Geometry: final body of the model. Coordinates: model frame, mm. Face numbers are marked on the shaded views. A direction names the side the tool comes from. Round coordinates to 2 decimals unless told otherwise and drop trailing zeros. Write each loop counter-clockwise with the first axis right and the second up, starting at its lowest first coordinate (ties: lowest second). Pieces come first, ordered by that corner, then holes.
from build123d import *

# Parameters (mm, degrees)
F0_W     = 12.7
F0_H     = 25.4
F1_DEPTH = 25.4
F3_W     = 12.7
F3_H     = 12.7
F4_DEPTH = 6.35
F5_W     = 12.7
F5_H     = 25.4
F6_DEPTH = 12.7


with BuildPart() as f1:
    # F0 (on Front) → F1 (new body)
    with BuildSketch(Plane.XZ):
        with Locations((6.35, 12.7)):
            Rectangle(F0_W, F0_H)
    extrude(amount=-F1_DEPTH)

    # F3 (on face) → F4 (cut)
    with BuildSketch(Plane.XZ):
        with Locations((6.35, 12.7)):
            Rectangle(F3_W, F3_H)
    extrude(amount=-F4_DEPTH, mode=Mode.SUBTRACT)

    # F5 (on face) → F6 (join)
    with BuildSketch(Plane.YZ.offset(12.7)):
        with Locations((19.05, 12.7)):
            Rectangle(F5_W, F5_H)
    extrude(amount=F6_DEPTH)


solid = f1.part
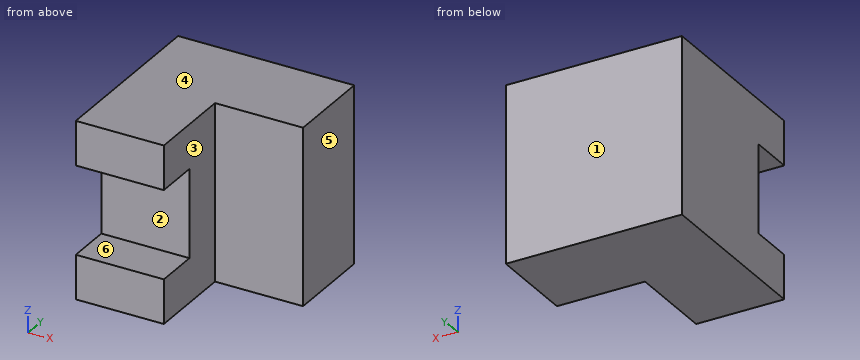
1) Section D-D on y = 12.25. Output: boundary loops of the cut face in (x, z).
2) First-contact query: P1, Ø10, axis at x = 14.5, y = 18, coming from the -Z side; P2, Ø2, axis at x = 17.5, z = 14.5, coming from the -Y side; P3, Ø6.5, axis at y = 4.5, z = 16, coming from the +X side; P4, Ø6.5, axis at x = 9.5, z = 15, coming from the -Y side. Flat tips, straight axial feed; report the tip coordinate or a pass-through.
3) Section C-C on z = 3.75. Output: boundary loops of the cut face in (x, y), plus the area to 3 significant figures.
4) Draft query along Z for the marked faces 4, 5 and 6. Return one class per face: pulls with the +Z half, pulls with the -Z half, needs draft (parallel to the pull), parting line crosses it, or undercut.
5) Line query: probe 1 along Z at (x, y) = (4, 3.5); probe 2 along Y at (x, z) = (6.25, 8); probe 3 along Y at (x, z) = (18.5, 3). Output: solid intervals per line, ascending.
6) Section B-B on x = 11.5. Output: boundary loops of the cut face in (y, z), plus the area to 3 significant figures.
7) Section A-A on y = 2. Output: boundary loops of the cut face in (x, z).
8) Reachability of the marked faces 1, 2 and 3 from +Z, -Z, +X, -X, +Y, -Y: full face, straight path, thin tool, end or side. Return the list, or none.
Filled in:
1. outline: (0, 0) - (12.7, 0) - (12.7, 25.4) - (0, 25.4) - close
2. P1: stops at z = 0
2. P2: stops at y = 12.7
2. P3: stops at x = 12.7
2. P4: stops at y = 6.35
3. outline: (0, 0) - (12.7, 0) - (12.7, 12.7) - (25.4, 12.7) - (25.4, 25.4) - (0, 25.4) - close
3. area: 484 mm2
4. face 4: pulls with the +Z half
4. face 5: needs draft
4. face 6: undercut
5. probe 1: z = 0 to 6.35, 19.05 to 25.4
5. probe 2: y = 6.35 to 25.4
5. probe 3: y = 12.7 to 25.4
6. outline: (0, 0) - (25.4, 0) - (25.4, 25.4) - (0, 25.4) - (0, 19.05) - (6.35, 19.05) - (6.35, 6.35) - (0, 6.35) - close
6. area: 565 mm2
7. outline: (0, 0) - (12.7, 0) - (12.7, 6.35) - (0, 6.35) - close; (0, 19.05) - (12.7, 19.05) - (12.7, 25.4) - (0, 25.4) - close
8. face 1: +Z, -Z, +X, -X, +Y
8. face 2: +X, -X, -Y
8. face 3: +Z, -Z, +X, -Y
